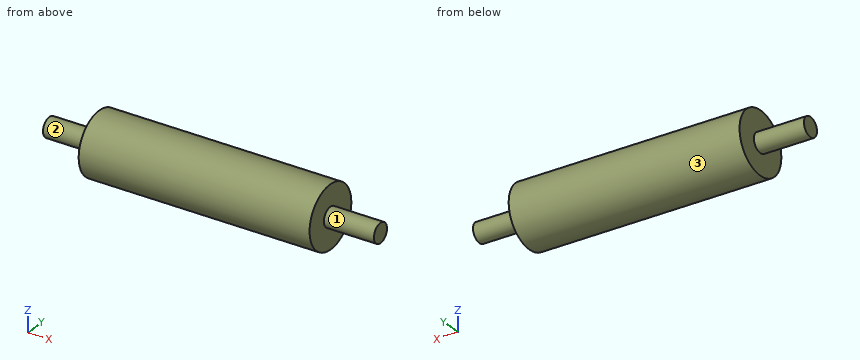
from build123d import *

# Parameters (mm, degrees)
SKETCH1_R           = 8
BOSS_EXTRUDE1_DEPTH = 30
SKETCH2_R           = 2.5
BOSS_EXTRUDE2_DEPTH = 13


with BuildPart() as part:
    # Sketch1 → Boss-Extrude1 (new body)
    with BuildSketch(Plane(origin=(0, 0, 0), x_dir=(0, 0, -1), z_dir=(1, 0, 0))):
        Circle(SKETCH1_R)
    boss_extrude1 = extrude(amount=BOSS_EXTRUDE1_DEPTH)

    # Sketch2 → Boss-Extrude2 (add)
    with BuildSketch(Plane(origin=(30, 0, 0), x_dir=(0, 0, -1), z_dir=(1, 0, 0))):
        with Locations(Location((0, 0, 0), (0, 0, 180))):
            Circle(SKETCH2_R)
    boss_extrude2 = extrude(amount=BOSS_EXTRUDE2_DEPTH)

    # Mirror1: Boss-Extrude1, Boss-Extrude2 across plane
    add(boss_extrude1.mirror(Plane(origin=(0, 0, 0), x_dir=(0, 0, 1), z_dir=(1, 0, 0))))
    add(boss_extrude2.mirror(Plane(origin=(0, 0, 0), x_dir=(0, 0, 1), z_dir=(1, 0, 0))))


solid = part.part
The listing builds one solid part. Answer for the finished solid, in the listing's coordinates (mm). Face numbers are marked on the shaded views. A direction names the side the tool comes from. Round coordinates to 2 decimals unless told otherwise and drop trailing zeros. Order: outer loops, then holes, each group sorted by start corner. A loop starts at its lowest first (then second) coordinate and runs counter-clockwise, first axis right, second up. Notation, with made-up numbers: (36.25, -18.5) - (45.25, -18.5) arc R13 cw to (45.25, -3.5) - close; hole circle Ø1 at (74.25, 74.5). An arc over 180 degrees is marked (long way). Write item = value, one per line. Start each with the question number.
1) Straight lines are drawn through the part: L1, parallel to X at y = -5.5, z = 5.25; L2, parallel to Z at x = 9, y = 2.75; L3, parallel to Y at x = 2.5, z = -4. For each, find the intervals that lie inside material, in ascending order.
2) Section C-C, the plane x = 34.5 is taken. Write down the section's boundary in (y, z).
3) Given pin 1 (2 mm diameter, centred on y = -1, z = 5.5, fed in from -X); pin 2 (1.5 mm diameter, centred on x = 1.5, y = 2, fed in from -Z); pin 3 (3 mm diameter, centred on x = 30.5, y = 2.5, fed in from +Z), each flat-ended and moving along its own axis, determine where each tip first touches the part or whether it passes through.
4) For the marked faces 1, 2 and 3, determine the directions among +Z, -Z, +X, -X, +Y, -Y from which every point of the face is accessible in a straight line to the end or side of a thin tool.
5) Section D-D, the plane x = 14.5 is taken. Write down the section's boundary in (y, z).
6) Section A-A, the plane y = 0 is taken. Write down the section's boundary in (x, z), plus the area to 3 significant figures.
Results list:
q1.L1 = -30 to 30
q1.L2 = -7.51 to 7.51
q1.L3 = -6.93 to 6.93
q2.outline = circle Ø5 at (0, 0)
q3.pin_1 = -30
q3.pin_2 = -7.9
q3.pin_3 = 7.93
q4.face_1 = +X
q4.face_2 = -X
q4.face_3 = +X, -X
q5.outline = circle Ø16 at (0, 0)
q6.outline = (-43, -2.5) - (-30, -2.5) - (-30, -8) - (30, -8) - (30, -2.5) - (43, -2.5) - (43, 2.5) - (30, 2.5) - (30, 8) - (-30, 8) - (-30, 2.5) - (-43, 2.5) - close
q6.area = 1,090 mm^2
